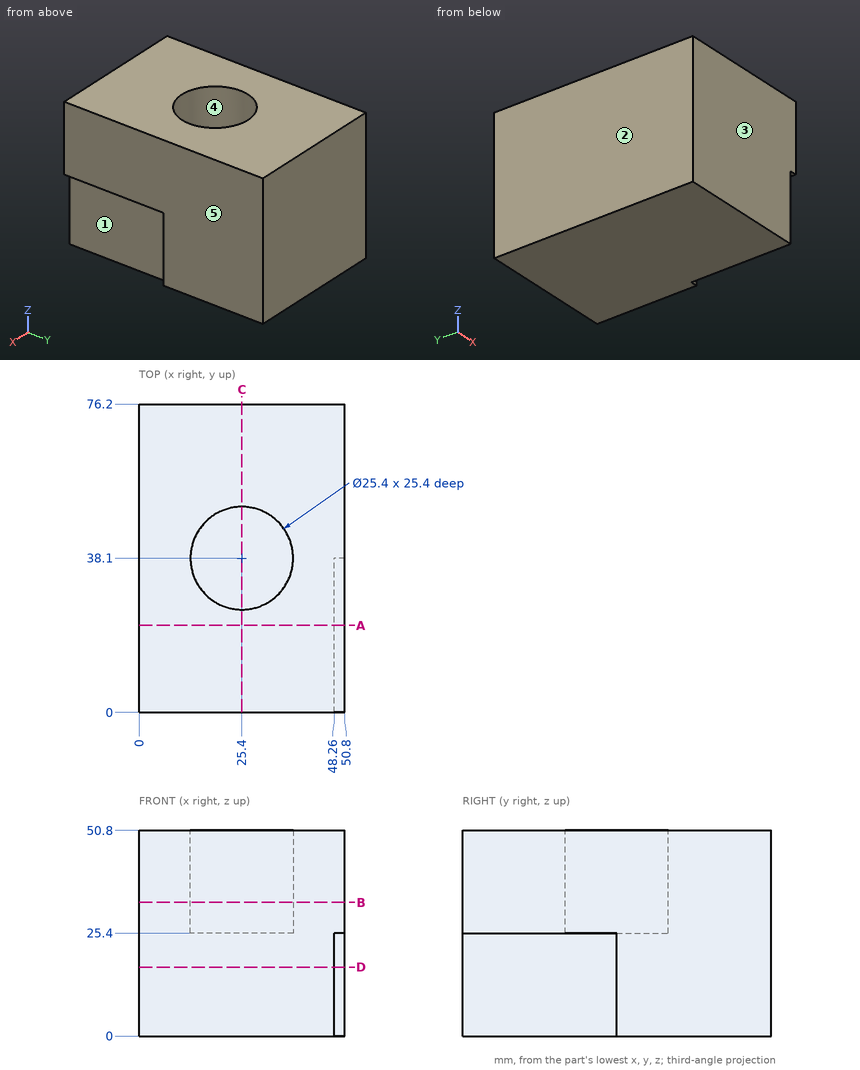
Verification items for this drawing (mm, ordinates from the low corner). A direction names the side the tool comes from. Give positions to 0.01 mm unless a question says otherwise; leave off trailing zeros. Loops run counter-clockwise (first coordinate to the right, second up) from the corner with the lowest first, then second, coordinate; pieces in that order, holes last. Notation, with made-up numbers: M -20.75,-29 L 19.25,-29 A16 cw 19.25,-17 Z; hole C 88.25,39.5 d5. An arc over 180 degrees is marked long. Write each question's results on one line, items separated by ' | '.
1) Section check A-A, the plane y = 21.5. Record the boundary of the cut face in (x, z).
Answers follow:
outline: M 0,0 L 48.26,0 L 48.26,25.4 L 50.8,25.4 L 50.8,50.8 L 0,50.8 Z
2) Section check B-B, the plane z = 33. Record the boundary of the cut face in (x, y).
Answers follow:
outline: M 0,0 L 50.8,0 L 50.8,76.2 L 0,76.2 Z; hole C 25.4,38.1 d25.4
3) Thickness scan on line 1 (Y direction, x = 25, z = 41); line 2 (X direction, y = 38, z = 40); line 3 (X direction, y = 48, z = 37). Record the ranges inside material, lowest first.
Answers follow:
line 1: 0 to 25.41, 50.79 to 76.2 | line 2: 0 to 12.7, 38.1 to 50.8 | line 3: 0 to 17.45, 33.35 to 50.8
4) Section check D-D, the plane z = 17. Record the boundary of the cut face in (x, y).
Answers follow:
outline: M 0,0 L 48.26,0 L 48.26,38.1 L 50.8,38.1 L 50.8,76.2 L 0,76.2 Z
5) Gauge pin test, flat ends, axial feed: pin 1 (0.8 mm diameter, centred on x = 49.5, z = 7.5, fed in from -Y); pin 2 (5 mm diameter, centred on y = 18.5, z = 9, fed in from +X). Record the tip position at first contact, or that the pin passes through.
Answers follow:
pin 1: y = 38.1 | pin 2: x = 48.26
6) Tool access check on the marked faces 1 and 2. Record the directions out of +Z, -Z, +X, -X, +Y, -Y that give a thin tool (end or side, any length) a straight path to the whole face; none if there is none.
Answers follow:
face 1: -Z, +X, -Y | face 2: +Z, -Z, -X, +Y, -Y
7) Release check for a two-part mould opening along X. For the marked faces 3, 4 and 5 record: +X half, -X half, draft (parallel to the pull), parting line (faces both ways), or undercut.
Answers follow:
face 3: draft | face 4: undercut | face 5: +X half
8) Section check C-C, the plane x = 25.4. Record the boundary of the cut face in (y, z), plus the area to 3 significant figures.
Answers follow:
outline: M 0,0 L 76.2,0 L 76.2,50.8 L 50.8,50.8 L 50.8,25.4 L 25.4,25.4 L 25.4,50.8 L 0,50.8 Z | area: 3,230 mm2
